Job drawing, mm, ordinate dimensions from the low corner. One solid piece. A direction names the side the tool comes from. Give positions to 0.01 mm unless a question says otherwise; leave off trailing zeros. Write each loop counter-clockwise with the first axis right and the second up, starting at its lowest first coordinate (ties: lowest second). Pieces come first, ordered by that corner, then holes. Notation, with made-up numbers: (58, 49) - (85, 49) arc R10 ccw to (85, 57) - close; hole circle Ø8 at (15, 32). An arc over 180 degrees is marked (long way). Answer in a Markdown table with one row per item. Add a question column.
1. Band-saw the part on C-C on x = 14. Write the cut outline in (y, z), plus the area to 3 significant figures.
2. Band-saw the part on B-B on z = 1.5. State how many separate pieces and enclosed holes the cut face has, plus the area to 3 significant figures.
3. Probe line 1 along Y through (x, z) = (10.5, 1.3); line 2 along Y through (x, z) = (13.75, 0.75); line 3 along Y through (x, z) = (18.8, 2). List the from-to ranges inside material, lowest first.
4. Which spindle directions (+Z, -Z, +X, -X, +Y, -Y) get a long thin tool onto all of the face, cutting with end or side? Do the marked faces 4 and 5. Say none if no direction does.
5. Band-saw the part on D-D on y = 6.75. Write the cut outline in (x, z), plus the area to 3 significant figures.
6. Drop flat-ended pins along their axis: pin 1 Ø2.5 at (x, y) = (18.8, 10.5) entering from -Z; pin 2 Ø1.8 at (x, y) = (10.5, 2.2) entering from +Z; pin 3 Ø3 at (y, z) = (13, 2.5) entering from +X. Give the stop position or say it passes through.
7. Band-saw the part on A-A on x = 10.5. Write the cut outline in (y, z), plus the area to 3 significant figures.
8. Pull direction X, two halves, no side cores. Call the marked faces 1, 2 and 3: released by +X, released by -X, zero draft, split by the parting line, or undercut.
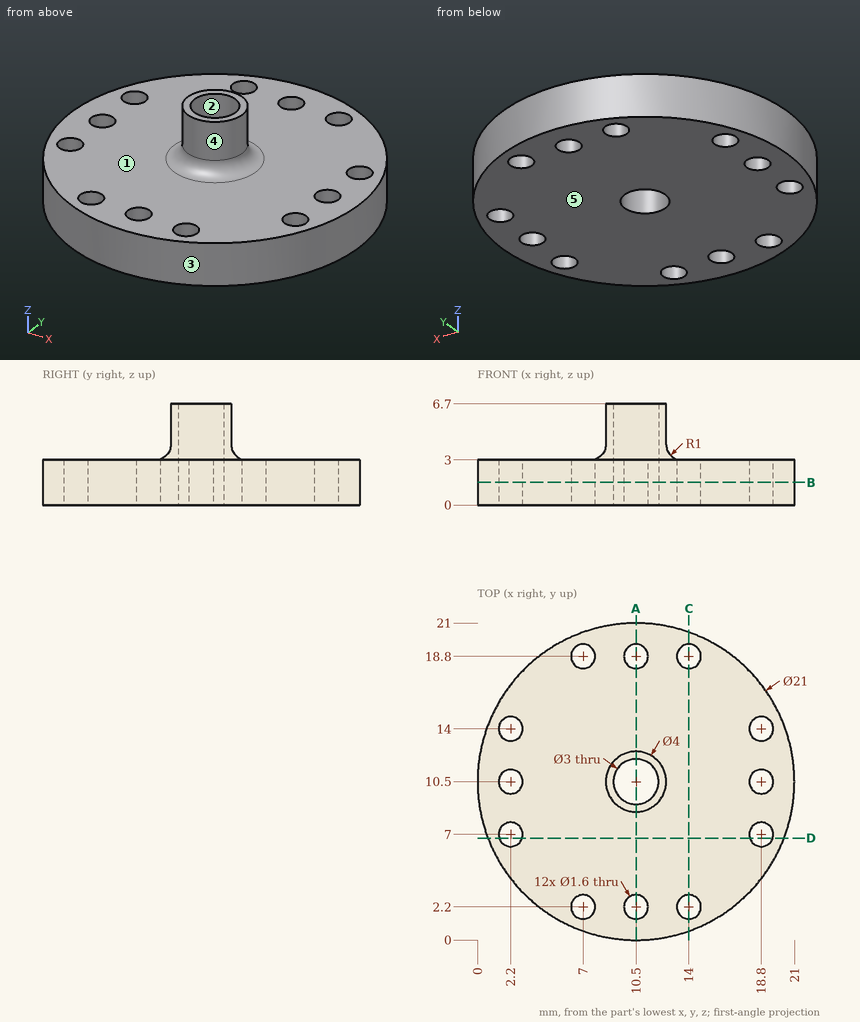
Values:
| question | item | result |
|---|---|---|
| 1 | outline | (0.6, 0) - (1.4, 0) - (1.4, 3) - (0.6, 3) - close; (3, 0) - (18, 0) - (18, 3) - (3, 3) - close; (19.6, 0) - (20.4, 0) - (20.4, 3) - (19.6, 3) - close |
| 1 | area | 49.8 mm² |
| 2 | separate pieces | 1 |
| 2 | enclosed holes | 13 |
| 2 | area | 315 mm² |
| 3 | line 1 | y = 0 to 1.4, 3 to 9, 12 to 18, 19.6 to 21 |
| 3 | line 2 | y = 0.52 to 1.44, 2.96 to 18.04, 19.56 to 20.48 |
| 3 | line 3 | y = 4.07 to 6.2, 7.8 to 9.7, 11.3 to 13.2, 14.8 to 16.93 |
| 4 | face 4 | +Z |
| 4 | face 5 | -Z, +X, -X, +Y, -Y |
| 5 | outline | (0.69, 0) - (1.44, 0) - (1.44, 3) - (0.69, 3) - close; (2.96, 0) - (18.04, 0) - (18.04, 3) - (2.96, 3) - close; (19.56, 0) - (20.31, 0) - (20.31, 3) - (19.56, 3) - close |
| 5 | area | 49.7 mm² |
| 6 | pin 1 | stops at z = 0 |
| 6 | pin 2 | stops at z = 3 |
| 6 | pin 3 | stops at x = 20.95 |
| 7 | outline | (0, 0) - (1.4, 0) - (1.4, 3) - (0, 3) - close; (3, 0) - (9, 0) - (9, 6.7) - (8.5, 6.7) - (8.5, 4) arc R1 cw to (7.5, 3) - (3, 3) - close; (12, 0) - (18, 0) - (18, 3) - (13.5, 3) arc R1 cw to (12.5, 4) - (12.5, 6.7) - (12, 6.7) - close; (19.6, 0) - (21, 0) - (21, 3) - (19.6, 3) - close |
| 7 | area | 48.5 mm² |
| 8 | face 1 | zero draft |
| 8 | face 2 | undercut |
| 8 | face 3 | split by the parting line |
